from build123d import *

# Parameters (mm, degrees)
BOSS_EXTRUDE1_DEPTH = 2.5
SKETCH2_R           = 1
CUT_EXTRUDE1_DEPTH  = 23.231734075


with BuildPart() as part:
    # Sketch1 → Boss-Extrude1 (new body)
    with BuildSketch(Plane(origin=(0, 0, 0), x_dir=(1, 0, 0), z_dir=(0, 1, 0))):
        with BuildLine():
            ThreePointArc((-20, 2), (-22, 0), (-20, -2))
            Line((-20, -2), (-20, 2))
        make_face()
        with BuildLine():
            Line((-20, 2), (-20, -2))
            ThreePointArc((-20, -2), (-18.585786438, -1.414213562), (-18, 0))
            ThreePointArc((-18, 0), (-18.585786438, 1.414213562), (-20, 2))
        make_face()
        with BuildLine():
            ThreePointArc((-18, 0), (-18.585786438, -1.414213562), (-20, -2))
            Line((-20, -2), (20, -2))
            ThreePointArc((20, -2), (18, 0), (20, 2))
            Line((20, 2), (-20, 2))
            ThreePointArc((-20, 2), (-18.585786438, 1.414213562), (-18, 0))
        make_face()
        with BuildLine():
            ThreePointArc((20, 2), (18, 0), (20, -2))
            Line((20, -2), (20, 2))
        make_face()
        with BuildLine():
            Line((20, 2), (20, -2))
            ThreePointArc((20, -2), (21.414213562, -1.414213562), (22, 0))
            ThreePointArc((22, 0), (21.414213562, 1.414213562), (20, 2))
        make_face()
    extrude(amount=BOSS_EXTRUDE1_DEPTH)

    # Sketch2 → Cut-Extrude1 (cut, through all)
    with BuildSketch(Plane(origin=(0, 0, 0), x_dir=(1, 0, 0), z_dir=(0, 1, 0))):
        with Locations(Location((20, 0, 0), (0, 0, 270))):
            Circle(SKETCH2_R)
        with Locations(Location((-20, 0, 0), (0, 0, 270))):
            Circle(SKETCH2_R)
    extrude(amount=CUT_EXTRUDE1_DEPTH, mode=Mode.SUBTRACT)


solid = part.part
For this review, take the finished solid that the model builds, in its own axes (mm). Round coordinates to 2 decimals unless told otherwise and drop trailing zeros. Order: outer loops, then holes, each group sorted by start corner. A loop starts at its lowest first (then second) coordinate and runs counter-clockwise, first axis right, second up. Notation, with made-up numbers: (-8.5, -32) -> (41.5, -32) arc R30 ccw to (41.5, 3) -> close; hole circle Ø5 at (-37.5, 68.25). An arc over 180 degrees is marked (long way). Write item = value, one per line. Start each with the question number.
1) Take a section at A-A on y = 1.75. State the section outline as (x, z) points, plus the area to 3 significant figures.
2) Take a section at B-B on z = 1.45. State the section outline as (x, y) points.
3) Insertion check: pin 1 (1 mm diameter, centred on y = 1.5, z = 1.5, fed in from -X); pin 2 (1.8 mm diameter, centred on x = 20, z = 0, fed in from -Y). Each pin has a flat end and moves straight along its axis. Give the tip position at first contact, or say it passes through.
4) The part is to be moulded in two halves that separate along Z. For faces 1 (the face through (-22, 1, 0)), 2 (the face through (19, 1, 0)), 3 (the face through (-21, 1, 0)), 4 (the face through (0, 0, 0)), say which applies: +Z half, -Z half, draft (parallel to the pull), parting line (faces both ways), or undercut.
5) To check wall thickness, follow line 1 (X direction, y = 0.3, z = -0.3); line 2 (Z direction, x = 20, y = 1.5); line 3 (X direction, y = 0.75, z = -0.8). State the ranges of each line that lie inside material, in increasing order. Write a range as from..to.
Verdict:
q1.outline = (-20, -2) -> (20, -2) arc R2 ccw to (20, 2) -> (-20, 2) arc R2 ccw to start; hole circle Ø2 at (-20, 0); hole circle Ø2 at (20, 0)
q1.area = 166 mm2
q2.outline = (-21.38, 0) -> (21.38, 0) -> (21.38, 2.5) -> (-21.38, 2.5) -> close
q3.pin_1 = -21.73
q3.pin_2 = through
q4.face_1 = parting line
q4.face_2 = undercut
q4.face_3 = undercut
q4.face_4 = draft
q5.line_1 = -21.98..-20.95, -19.05..19.05, 20.95..21.98
q5.line_2 = -2..-1, 1..2
q5.line_3 = -21.83..-20.6, -19.4..19.4, 20.6..21.83
